The figure shows three views and two pictorial views of one solid part (mm, origin at its lowest corner). Answer the questions. Round coordinates to 2 decimals unless told otherwise and drop trailing zeros. Order: outer loops, then holes, each group sorted by start corner. A loop starts at its lowest first (then second) coordinate and runs counter-clockwise, first axis right, second up. Notation, with made-up numbers: (53.5, -1) - (104.5, -1) arc R27 cw to (104.5, 26) - close; hole circle Ø3 at (-24, -15). An arc over 180 degrees is marked (long way). Answer in a Markdown table with one row per item.
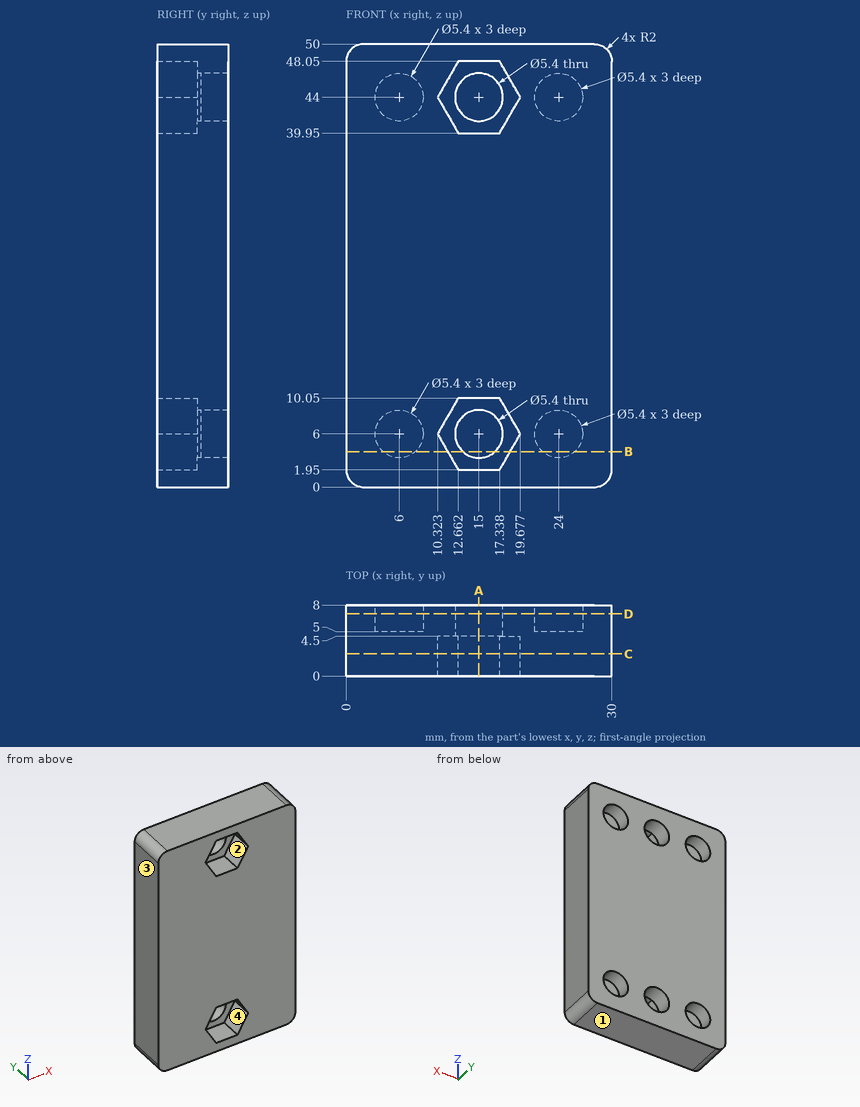
1) The mould has two halves that part along X. Classify the marked faces 1, 2, 3 and 4: released by +X, released by -X, zero draft, split by the parting line, or undercut.
Filled in:
| item | result |
|---|---|
| face 1 | zero draft |
| face 2 | undercut |
| face 3 | released by -X |
| face 4 | undercut |
2) Find section C-C, the plane y = 2.5. Give the vertices of the cut face in (x, z).
Filled in:
| item | result |
|---|---|
| outline | (0, 2) arc R2 ccw to (2, 0) - (28, 0) arc R2 ccw to (30, 2) - (30, 48) arc R2 ccw to (28, 50) - (2, 50) arc R2 ccw to (0, 48) - close; hole (10.32, 6) - (12.66, 1.95) - (17.34, 1.95) - (19.68, 6) - (17.34, 10.05) - (12.66, 10.05) - close; hole (10.32, 44) - (12.66, 39.95) - (17.34, 39.95) - (19.68, 44) - (17.34, 48.05) - (12.66, 48.05) - close |
3) Find section A-A, the plane x = 15. Give the vertices of the cut face in (y, z).
Filled in:
| item | result |
|---|---|
| outline | (0, 0) - (8, 0) - (8, 3.3) - (4.5, 3.3) - (4.5, 1.95) - (0, 1.95) - close; (0, 10.05) - (4.5, 10.05) - (4.5, 8.7) - (8, 8.7) - (8, 41.3) - (4.5, 41.3) - (4.5, 39.95) - (0, 39.95) - close; (0, 48.05) - (4.5, 48.05) - (4.5, 46.7) - (8, 46.7) - (8, 50) - (0, 50) - close |
4) Find the intervals of material crossed by probe 1 along Z at (x, y) = (6, 7.1); probe 2 along Z at (x, y) = (17.5, 3.5); probe 3 along X at (y, z) = (2, 45.5), in increasing order. Write a range as from..to.
Filled in:
| item | result |
|---|---|
| probe 1 | z = 0..3.3, 8.7..41.3, 46.7..50 |
| probe 2 | z = 0..2.23, 9.77..40.23, 47.77..50 |
| probe 3 | x = 0..11.19, 18.81..30 |
5) Find section D-D, the plane y = 7. Give the vertices of the cut face in (x, z), then the cut area to 3 significant figures.
Filled in:
| item | result |
|---|---|
| outline | (0, 2) arc R2 ccw to (2, 0) - (28, 0) arc R2 ccw to (30, 2) - (30, 48) arc R2 ccw to (28, 50) - (2, 50) arc R2 ccw to (0, 48) - close; hole circle Ø5.4 at (6, 6); hole circle Ø5.4 at (6, 44); hole circle Ø5.4 at (15, 6); hole circle Ø5.4 at (15, 44); hole circle Ø5.4 at (24, 6); hole circle Ø5.4 at (24, 44) |
| area | 1,360 mm^2 |
6) Each of these flat-tipped pins is pushed along its axis until it touches: pin 1 (7 mm diameter, centred on x = 6, z = 6, fed in from -Y); pin 2 (5 mm diameter, centred on x = 15, z = 6, fed in from +Y); pin 3 (1.6 mm diameter, centred on x = 5, z = 43.5, fed in from +Y). Where does it stop, or does it pass through?
Filled in:
| item | result |
|---|---|
| pin 1 | stops at y = 0 |
| pin 2 | passes through |
| pin 3 | stops at y = 5 |
7) Find section B-B, the plane z = 4. Give the vertices of the cut face in (x, y).
Filled in:
| item | result |
|---|---|
| outline | (0, 0) - (11.48, 0) - (11.48, 4.5) - (13.19, 4.5) - (13.19, 8) - (7.81, 8) - (7.81, 5) - (4.19, 5) - (4.19, 8) - (0, 8) - close; (16.81, 4.5) - (18.52, 4.5) - (18.52, 0) - (30, 0) - (30, 8) - (25.81, 8) - (25.81, 5) - (22.19, 5) - (22.19, 8) - (16.81, 8) - close |
